```python
from build123d import *

# Parameters (mm, degrees)
PAD_DEPTH            = 25
FILLET_R             = 5
SKETCH001_R          = 2
SKETCH001_R_2        = 1.5
POCKET_DEPTH         = 12.501
POCKET_DEPTH_BACK    = -12.501
FILLET001_R          = 1
BODY_PLACEMENT_ANGLE = 270


with BuildPart() as part:
    # Sketch → Pad (new body, symmetric)
    with BuildSketch(Plane.XY):
        Polygon((-12.5, 1), (-12.5, -1), (12.5, -1), (12.5, 1), (1, 1), (1, 141), (-1, 141), (-1, 1), align=None)
    extrude(amount=PAD_DEPTH, both=True)

    # Fillet
    fillet_edges = [part.edges().sort_by_distance(p)[0] for p in [
        (-1, 1, 0),
        (1, 1, 0),
    ]]
    fillet(fillet_edges, radius=FILLET_R)

    # Sketch001 → Pocket (cut, two sides)
    with BuildSketch(Plane.YZ) as pocket_sk:
        with Locations((135.847954, 20)):
            Circle(SKETCH001_R)
        with Locations((95.847954, -20)):
            Circle(SKETCH001_R)
        with Locations((9.567412, 14.346174)):
            Circle(SKETCH001_R_2)
        with Locations((16.322672, 18.952028)):
            Circle(SKETCH001_R_2)
    extrude(amount=-POCKET_DEPTH, mode=Mode.SUBTRACT)
    extrude(pocket_sk.sketch, amount=-POCKET_DEPTH_BACK, mode=Mode.SUBTRACT)

    # Fillet001
    fillet001_edges = [part.edges().sort_by_distance(p)[0] for p in [
        (-12.5, 1, 0),
        (12.5, 1, 0),
    ]]
    fillet(fillet001_edges, radius=FILLET001_R)


with BuildPart() as part_1:
    # Body placement: moved
    add(part.part.rotate(Axis((0, 0, 0), (0, 1, 0)), BODY_PLACEMENT_ANGLE))


solid = part_1.part
```
Build history of the part. All positions in model axes, mm. A direction names the side the tool comes from. Round coordinates to 2 decimals unless told otherwise and drop trailing zeros. Write each loop counter-clockwise with the first axis right and the second up, starting at its lowest first coordinate (ties: lowest second). Pieces come first, ordered by that corner, then holes.
1) Pin check, flat tips, straight feed: pin 1 (5 mm diameter, centred on x = -20, y = 135.85, fed in from +Z); pin 2 (2 mm diameter, centred on x = 8.5, z = -5, fed in from +Y); pin 3 (25 mm diameter, centred on x = -2.5, y = 85.5, fed in from -Z). Stop position of each tip, or through.
2) Band-saw the part on D-D, the plane x = 13.5. List the corners of the cut face in (y, z).
3) Band-saw the part on B-B, the plane y = 117.5. List the corners of the cut face in (x, z), and give its area (3 significant figures).
4) 3-axis set-ups, long thin cutter, end or side, ignore diameter. For faces 1 (the flat face through (0, 73, 1)), 2 (the flat face through (0, 74, -1)), 3 (the flat face through (0, -1, 0)): which of +Z, -Z, +X, -X, +Y, -Y reach the whole face in a straight line?
5) Band-saw the part on A-A, the plane x = 20. List the corners of the cut face in (y, z).
6) Drill centre lines: probe 1 along Y at (x, z) = (-20, -0.7); probe 2 along Y at (x, z) = (20, 0.4); probe 3 along Z at (x, y) = (9, 26). Where is each one in solid material? Low to high.
Ans:
1. pin 1: stops at z = 1
1. pin 2: stops at y = 1.42
1. pin 3: stops at z = -1
2. outline: (-1, -12.5) - (0, -12.5) arc R1 ccw to (1, -11.5) - (1, -6) arc R5 cw to (6, -1) - (141, -1) - (141, 1) - (6, 1) arc R5 cw to (1, 6) - (1, 11.5) arc R1 ccw to (0, 12.5) - (-1, 12.5) - close
3. outline: (-25, -1) - (25, -1) - (25, 1) - (-25, 1) - close
3. area: 100 mm2
4. face 1: +Z, +X, -X, +Y
4. face 2: -Z, +X, -X, +Y
4. face 3: +Z, -Z, +X, -X, -Y
5. outline: (-1, -12.5) - (0, -12.5) arc R1 ccw to (1, -11.5) - (1, -6) arc R5 cw to (6, -1) - (93.85, -1) - (93.85, 1) - (6, 1) arc R5 cw to (1, 6) - (1, 11.5) arc R1 ccw to (0, 12.5) - (-1, 12.5) - close; (97.85, -1) - (141, -1) - (141, 1) - (97.85, 1) - close
6. probe 1: y = -1 to 15.25, 17.4 to 133.85, 137.85 to 141
6. probe 2: y = -1 to 93.85, 97.85 to 141
6. probe 3: z = -1 to 1
